Model file for the job. Use its own axes, mm. Round coordinates to 2 decimals unless told otherwise and drop trailing zeros. Write each loop counter-clockwise with the first axis right and the second up, starting at its lowest first coordinate (ties: lowest second). Pieces come first, ordered by that corner, then holes.
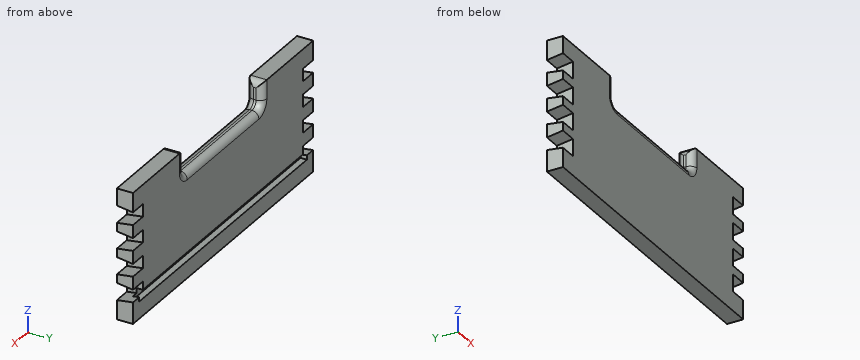
```python
from build123d import *

# Parameters (mm, degrees)
F0_W     = 230
F0_H     = 96.8045385678
F1_DEPTH = 12
F2_W     = 101.6
F2_H     = 19.05
F3_DEPTH = 12
F4_R     = 5.08
F6_DEPTH = 12.7
F7_W     = 204.6
F7_H     = 6.35
F7_W_2   = 4.7625
F8_DEPTH = 4.7625


# Not quite as in the source:
# - a pattern or mirror of a feature is missing from the dataset's text; its kind, count and spacing are read off the source's solid


with BuildPart() as f1:
    # F0 (on Front) → F1 (new body)
    with BuildSketch(Plane.XZ):
        Rectangle(F0_W, F0_H)
    extrude(amount=-F1_DEPTH)

    # F2 (on face) → F3 (cut, through all)
    with BuildSketch(Plane.XZ):
        with Locations((0, 38.8772692839)):
            Rectangle(F2_W, F2_H)
    extrude(amount=-F3_DEPTH, mode=Mode.SUBTRACT)

    # F4
    f4_edges = [f1.edges().sort_by_distance(p)[0] for p in [
        (-50.8, 6, 48.402269),
        (-50.8, 6, 29.352269),
        (-50.8, 0, 38.877269),
        (-50.8, 12, 38.877269),
        (50.8, 6, 29.352269),
        (50.8, 6, 48.402269),
        (50.8, 0, 38.877269),
        (50.8, 12, 38.877269),
        (0, 0, 29.352269),
        (0, 12, 29.352269),
    ]]
    fillet(f4_edges, radius=F4_R)

    # F5 (on face) → F6 (cut)
    with BuildSketch(Plane.YZ.offset(115)):
        Polygon((12, 34.0157792675), (0, 35.7022692839), (0, 23.0022692839), (12, 24.6887593003), align=None)
        Polygon((12, 14.9657792675), (0, 16.6522692839), (0, 3.9522692839), (12, 5.6387593003), align=None)
        Polygon((12, -4.0842207325), (0, -2.3977307161), (0, -15.0977307161), (12, -13.4112406997), align=None)
        Polygon((12, -23.1342207325), (0, -21.4477307161), (0, -34.1477307161), (12, -32.4612406997), align=None)
    f6 = extrude(amount=-F6_DEPTH, mode=Mode.SUBTRACT)

    # F6_copies: F6 across plane
    add(f6.mirror(Plane(origin=(0, 0, 0), x_dir=(0, 0, -1), z_dir=(-1, 0, 0))), mode=Mode.SUBTRACT)

    # F7 (on face) → F8 (cut)
    with BuildSketch(Plane(origin=(0, 12, 0), x_dir=(-1, 0, 0), z_dir=(0, 1, 0))):
        with Locations((0, -32.5272692839)):
            Rectangle(F7_W, F7_H)
        with Locations((-104.68125, -32.5272692839)):
            Rectangle(F7_W_2, F7_H)
        with Locations((104.68125, -32.5272692839)):
            Rectangle(F7_W_2, F7_H)
    extrude(amount=-F8_DEPTH, mode=Mode.SUBTRACT)


solid = f1.part
```
1) Wall check: probe 1 along X at (y, z) = (8.75, -34.5); probe 2 along Z at (x, y) = (-76.5, 8); probe 3 along X at (y, z) = (10.75, 14). Give the ranges that are in metal, low to high.
2) Cut at C-C on x = -70.5. List the corners of the cut face in (y, z), and give its area (3 significant figures).
3) Cut at A-A on x = 10. List the corners of the cut face in (y, z).
4) Flat gauge pins, fed straight in: pin 1 Ø0.6 at (x, y) = (-3.5, 6) entering from +Z; pin 2 Ø3.5 at (y, z) = (5.5, -24.5) entering from +X; pin 3 Ø5 at (x, z) = (28, -32) entering from +Y. Where does each tip first touch, or does it go through?
5) Cut at B-B on z = 10. List the corners of the cut face in (x, y), and give its area (3 significant figures).
Result sheet:
1. probe 1: x = -115 to -107.06, 107.06 to 115
1. probe 2: z = -48.4 to -35.7, -29.35 to 48.4
1. probe 3: x = -102.3 to 102.3
2. outline: (0, -48.4) - (12, -48.4) - (12, -35.7) - (7.24, -35.7) - (7.24, -29.35) - (12, -29.35) - (12, 48.4) - (0, 48.4) - close
2. area: 1,130 mm2
3. outline: (0, -48.4) - (12, -48.4) - (12, -35.7) - (7.24, -35.7) - (7.24, -29.35) - (12, -29.35) - (12, 24.27) arc R5.08 ccw to (6.92, 29.35) - (5.08, 29.35) arc R5.08 ccw to (0, 24.27) - close
4. pin 1: stops at z = 29.35
4. pin 2: stops at x = 102.3
4. pin 3: stops at y = 7.24
5. outline: (-102.3, 0) - (102.3, 0) - (102.3, 12) - (-102.3, 12) - close
5. area: 2,460 mm2
